Read the model definition and answer for the solid it produces. Units are mm, in the model's axes. A direction names the side the tool comes from. Coordinates: 2 decimals unless noted, no trailing zeros. Loops run counter-clockwise (first coordinate to the right, second up) from the corner with the lowest first, then second, coordinate; pieces in that order, holes last.
from build123d import *

# Parameters (mm, degrees)
EXTRUDE_1_DEPTH = 87
SKETCH_2_W      = 30.108921009
SKETCH_2_H      = 80.924328046


with BuildPart() as part:
    # 草图1 → 凸台-拉伸1 (new body)
    with BuildSketch(Plane.XY):
        with BuildLine():
            ThreePointArc((-20.80288439, 70.428851171), (-47.791271034, 69.651792293), (-58.226927057, 44.750508842))
            ThreePointArc((-58.226927057, 44.750508842), (-79.604246754, 28.258479352), (-73.41026265, 1.978993149))
            ThreePointArc((-73.41026265, 1.978993149), (-81.011105864, -23.928612231), (-60.553373033, -41.548430663))
            ThreePointArc((-60.553373033, -41.548430663), (-51.474476, -66.975787246), (-24.567153051, -69.205766141))
            ThreePointArc((-24.567153051, -69.205766141), (-2.276345856, -84.440487955), (20.80288439, -70.428851171))
            ThreePointArc((20.80288439, -70.428851171), (47.791271034, -69.651792293), (58.226927057, -44.750508842))
            ThreePointArc((58.226927057, -44.750508842), (79.604246754, -28.258479352), (73.41026265, -1.978993149))
            ThreePointArc((73.41026265, -1.978993149), (81.011105864, 23.928612231), (60.553373033, 41.548430663))
            ThreePointArc((60.553373033, 41.548430663), (51.474476, 66.975787246), (24.567153051, 69.205766141))
            ThreePointArc((24.567153051, 69.205766141), (2.276345856, 84.440487955), (-20.80288439, 70.428851171))
        make_face()
        with BuildLine():
            ThreePointArc((-11.286570005, 38.211054977), (0.933445053, 34.625913967), (13.328867648, 37.547472247))
            ThreePointArc((13.328867648, 37.547472247), (21.107774488, 27.464287609), (32.853130891, 22.542031311))
            ThreePointArc((32.853130891, 22.542031311), (33.219651496, 9.812236861), (39.82861477, -1.073699411))
            ThreePointArc((39.82861477, -1.073699411), (32.642750726, -11.587754862), (31.590921532, -24.279313452))
            ThreePointArc((31.590921532, -24.279313452), (19.597428665, -28.561618081), (11.286570005, -38.211054977))
            ThreePointArc((11.286570005, -38.211054977), (-0.933445053, -34.625913967), (-13.328867648, -37.547472247))
            ThreePointArc((-13.328867648, -37.547472247), (-21.107774488, -27.464287609), (-32.853130891, -22.542031311))
            ThreePointArc((-32.853130891, -22.542031311), (-33.219651496, -9.812236861), (-39.82861477, 1.073699411))
            ThreePointArc((-39.82861477, 1.073699411), (-32.642750726, 11.587754862), (-31.590921532, 24.279313452))
            ThreePointArc((-31.590921532, 24.279313452), (-19.597428665, 28.561618081), (-11.286570005, 38.211054977))
        make_face(mode=Mode.SUBTRACT)
    extrude(amount=EXTRUDE_1_DEPTH)

    # 草图2 → 切除-旋转1 (revolve, cut)
    with BuildSketch(Plane(origin=(0, 0, 0), x_dir=(1, 0, 0), z_dir=(0, 1, 0))):
        with Locations((-48.966613642, -59.188332526)):
            Rectangle(SKETCH_2_W, SKETCH_2_H)
    revolve(axis=Axis((0, 0, 0), (0, 0, 1)), mode=Mode.SUBTRACT)


solid = part.part
Q1. A cutting plane is placed at A-A (y = -17). Give the vertices of the cut face in (x, z).
Findings below:
outline: (-82.03, 0) - (-32.2, 0) - (-32.2, 18.73) - (-61.72, 18.73) - (-61.72, 87) - (-82.03, 87) - close; (31.38, 0) - (80.87, 0) - (80.87, 87) - (61.72, 87) - (61.72, 18.73) - (31.38, 18.73) - close
Q2. A cutting plane is placed at C-C (z = 57). Give the vertices of the cut face in (x, y), then the cut area to 3 significant figures.
Findings below:
outline: (-73.41, 1.98) arc R24.92 ccw to (-60.55, -41.55) arc R24.92 ccw to (-24.57, -69.21) arc R24.92 ccw to (20.8, -70.43) arc R24.92 ccw to (58.23, -44.75) arc R24.92 ccw to (73.41, -1.98) arc R24.92 ccw to (60.55, 41.55) arc R24.92 ccw to (24.57, 69.21) arc R24.92 ccw to (-20.8, 70.43) arc R24.92 ccw to (-58.23, 44.75) arc R24.92 ccw to start; hole circle Ø128.04 at (0, 0)
area: 7,750 mm2
Q3. Determine the mould class of faces 1 (the face through (-13, 63, 87)), 2 (the face through (-2.676, -84.427, 42.891)), 3 (the face through (-33.169, -9.985, 9.232)) for opening direction Y: +Y half, -Y half, draft (parallel to the pull), parting line (faces both ways), or undercut.
Findings below:
face 1: draft
face 2: -Y half
face 3: undercut
Q4. Straight lines are drawn through the part: probe 1 along X at (y, z) = (24.5, 38.5); probe 2 along Y at (x, z) = (21, 53); probe 3 along Z at (x, y) = (34, -30). For each, find the intervals that lie inside material, in ascending order.
Findings below:
probe 1: x = -80.62 to -59.15, 59.15 to 80.83
probe 2: y = -70.55 to -60.48, 60.48 to 75.17
probe 3: z = 0 to 18.73
Q5. Which of the six approach directions +Z, -Z, +X, -X, +Y, -Y give full straight-line access (tool end or side, diameter ignored) to faces 4 (the face through (13.88, 62.5, 52.39)), 5 (the face through (-32.704, 11.418, 9.232))?
Findings below:
face 4: +Z
face 5: +Z, -Z
Q6. Flat-ended cylindrical pins translate along their axes: pin 1 Ø6 at (x, z) = (2.5, 28.5) entering from -Y (3 decimals); pin 2 Ø6 at (y, z) = (-16, 15.5) entering from +X; pin 3 Ø12 at (y, z) = (-59, 44.5) entering from +X; pin 4 Ø12 at (y, z) = (-22.5, 31.5) entering from -X. Find the tip coordinate at first contact, or state that the pin passes through.
Findings below:
pin 1: stops at y = -84.425
pin 2: stops at x = 81.02
pin 3: stops at x = 58.3
pin 4: stops at x = -82.03
Q7. A cutting plane is placed at D-D (y = 48). Give the vertices of the cut face in (x, z).
Findings below:
outline: (-58.59, 0) - (61.2, 0) - (61.2, 87) - (42.36, 87) - (42.36, 18.73) - (-42.36, 18.73) - (-42.36, 87) - (-58.59, 87) - close
Q8. A cutting plane is placed at B-B (x = 0). Give the vertices of the cut face in (y, z).
Findings below:
outline: (-84.4, 0) - (-34.67, 0) - (-34.67, 18.73) - (-64.02, 18.73) - (-64.02, 87) - (-84.4, 87) - close; (34.67, 0) - (84.4, 0) - (84.4, 87) - (64.02, 87) - (64.02, 18.73) - (34.67, 18.73) - close
